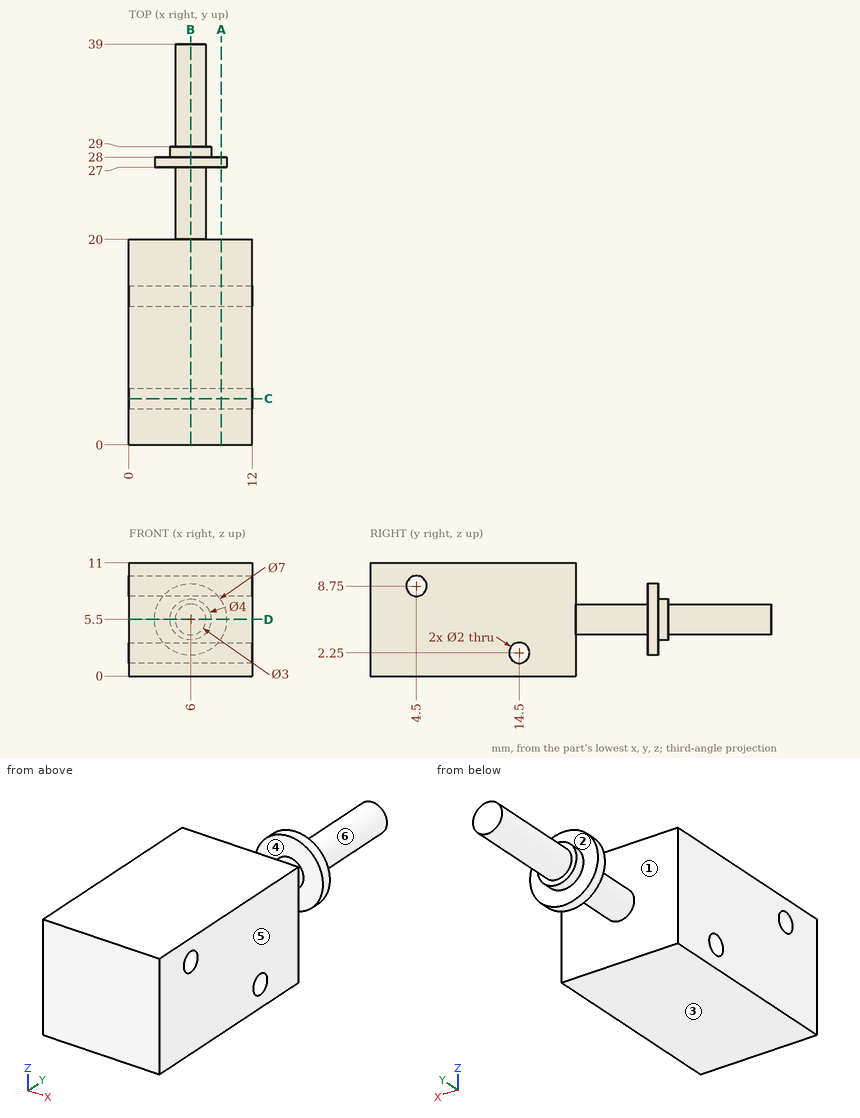
Here's the drawing with two shaded views (mm, measured from the low corner). I have some questions. A direction names the side the tool comes from. Give positions to 0.01 mm unless a question says otherwise; leave off trailing zeros. Write each loop counter-clockwise with the first axis right and the second up, starting at its lowest first coordinate (ties: lowest second). Pieces come first, ordered by that corner, then holes. Notation, with made-up numbers: (-19.5, 55.5) - (-2.5, 55.5) arc R25 cw to (-2.5, 74.5) - close; hole circle Ø5 at (-13, -7). An arc over 180 degrees is marked (long way). One line per item, written item: value. Start each with the question number.
Item 1: Imagine slicing it at B-B, the plane x = 6. List the corners of the cut face in (y, z) for me.
Item 2: Which directions (+Z, -Z, +X, -X, +Y, -Y) give clear straight access to the entire face, cutting with the end or side of a thin tool? Please do the marked faces 4, 5 and 6.
Item 3: Imagine slicing it at C-C, the plane y = 4.5. List the corners of the cut face in (x, z) for me, and give its area (3 significant figures).
Item 4: I'm going to push flat-ended pins straight in: pin 1 (4 mm diameter, centred on x = 3, z = 7, fed in from -Y); pin 2 (4 mm diameter, centred on x = 10.5, z = 5, fed in from +Y); pin 3 (1.8 mm diameter, centred on y = 4.5, z = 8.75, fed in from +X); pin 4 (6 mm diameter, centred on x = 6, y = 28, fed in from +Z). Where does each tip first touch, or does it pass through?
Item 5: If we mould it in two halves opening along Y, with no side actions, what happens to the marked faces 1, 2 and 3? For each: +Y half, -Y half, draft (parallel to the pull), parting line (faces both ways), or undercut.
Item 6: Please list where these lines run through material, in increasing order: line 1 (Y direction, x = 5.75, z = 2.25); line 2 (Y direction, x = 7.5, z = 8.75); line 3 (Y direction, x = 6, z = 3.75). Write a range as from..to.
Item 7: Imagine slicing it at A-A, the plane x = 9. List the corners of the cut face in (y, z) for me.
Item 8: Imagine slicing it at D-D, the plane z = 5.5. List the corners of the cut face in (x, y) for me, and give its area (3 significant figures).
Geometry says:
1. outline: (0, 0) - (20, 0) - (20, 4) - (27, 4) - (27, 2) - (28, 2) - (28, 3.5) - (29, 3.5) - (29, 4) - (39, 4) - (39, 7) - (29, 7) - (29, 7.5) - (28, 7.5) - (28, 9) - (27, 9) - (27, 7) - (20, 7) - (20, 11) - (0, 11) - close; hole circle Ø2 at (4.5, 8.75); hole circle Ø2 at (14.5, 2.25)
2. face 4: none
2. face 5: +Z, -Z, +X, +Y, -Y
2. face 6: +Y
3. outline: (0, 0) - (12, 0) - (12, 7.75) - (0, 7.75) - close; (0, 9.75) - (12, 9.75) - (12, 11) - (0, 11) - close
3. area: 108 mm^2
4. pin 1: y = 0
4. pin 2: y = 28
4. pin 3: through
4. pin 4: z = 9
5. face 1: undercut
5. face 2: +Y half
5. face 3: draft
6. line 1: 0..13.5, 15.5..20, 27..28
6. line 2: 0..3.5, 5.5..20
6. line 3: 0..20, 27..29
7. outline: (0, 0) - (20, 0) - (20, 11) - (0, 11) - close; (27, 3.7) - (28, 3.7) - (28, 7.3) - (27, 7.3) - close; hole circle Ø2 at (4.5, 8.75); hole circle Ø2 at (14.5, 2.25)
8. outline: (0, 0) - (12, 0) - (12, 20) - (7.5, 20) - (7.5, 27) - (9.5, 27) - (9.5, 28) - (8, 28) - (8, 29) - (7.5, 29) - (7.5, 39) - (4.5, 39) - (4.5, 29) - (4, 29) - (4, 28) - (2.5, 28) - (2.5, 27) - (4.5, 27) - (4.5, 20) - (0, 20) - close
8. area: 302 mm^2
